Check sheet for the drawn part. Datum: minimum x, y, z corner. Units: mm. A direction names the side the tool comes from. Round coordinates to 2 decimals unless told otherwise and drop trailing zeros. Write each loop counter-clockwise with the first axis right and the second up, starting at its lowest first coordinate (ties: lowest second). Pieces come first, ordered by that corner, then holes. Notation, with made-up numbers: (-27.5, 65) - (-9.5, 65) arc R24 ccw to (-9.5, 102) - close; hole circle Ø6 at (67, 71.25). An arc over 180 degrees is marked (long way). Answer as a JSON object with one key per item and string values. Group by question number.
1) Set-up check for the marked faces 1 and 2: record each of +Z, -Z, +X, -X, +Y, -Y from which the full face is reachable in a straight line by a thin tool's end or side.
2) Section check A-A (z = 3). Enter the section's corners in (x, y), then the cut area to 4 significant figures.
3) Thickness scan on line 1 (Y direction, x = 22.5, z = 16.25); line 2 (X direction, y = 2, z = 9.75). Record the ranges inside material, lowest first.
4) Go/stop test with flat-tipped pins: pin 1 Ø0.7 at (y, z) = (2.5, 8) entering from +X; pin 2 Ø2 at (x, z) = (22.5, 2) entering from +Y. Record where each tip stops, or that it passes through.
5) Section check C-C (x = 21). Enter the section's corners in (y, z), then the cut area to 4 significant figures.
6) Section check B-B (y = 2.7). Enter the section's corners in (x, z), then the cut area to 4 significant figures.
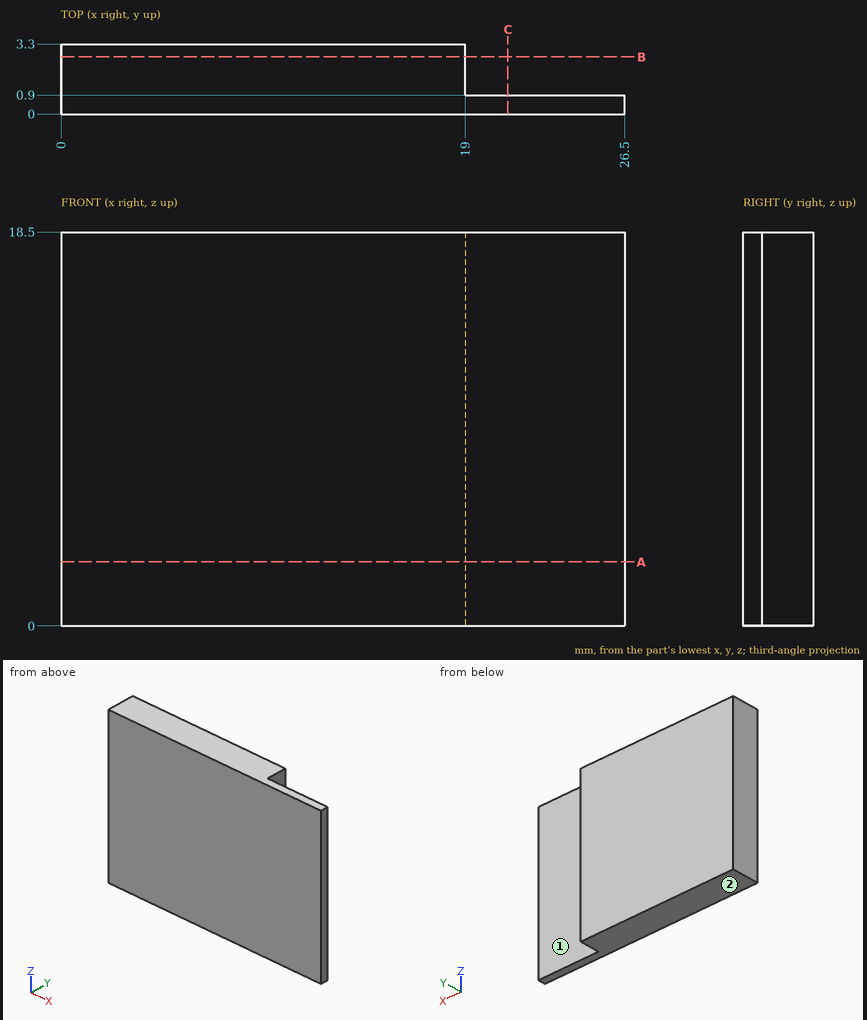
Returned:
{
 "1": {"face 1": "+Z, -Z, +X, +Y", "face 2": "-Z, +X, -X, +Y, -Y"},
 "2": {"outline": "(0, 0) - (26.5, 0) - (26.5, 0.9) - (19, 0.9) - (19, 3.3) - (0, 3.3) - close", "area": "69.45 mm2"},
 "3": {"line 1": "0 to 0.9", "line 2": "0 to 19"},
 "4": {"pin 1": "x = 19", "pin 2": "y = 0.9"},
 "5": {"outline": "(0, 0) - (0.9, 0) - (0.9, 18.5) - (0, 18.5) - close", "area": "16.65 mm2"},
 "6": {"outline": "(0, 0) - (19, 0) - (19, 18.5) - (0, 18.5) - close", "area": "351.5 mm2"}
}
